The listing builds one solid part. Answer for the finished solid, in the listing's coordinates (mm). A direction names the side the tool comes from. Coordinates: 2 decimals unless noted, no trailing zeros. Write each loop counter-clockwise with the first axis right and the second up, starting at its lowest first coordinate (ties: lowest second). Pieces come first, ordered by that corner, then holes. Notation, with made-up numbers: M -14,-19 L 33,-19 A11 ccw 33,-15 Z; hole C 22,-1.5 d6. An arc over 180 degrees is marked long. Put each result on its own line as item: value. Start each with the question number.
```python
from build123d import *

# Parameters (mm, degrees)
F0_W     = 26
F0_H     = 128
F1_DEPTH = 17
F2_W     = 4
F2_H     = 40
F3_DEPTH = 15
F4_R     = 1


with BuildPart() as f1:
    # F0 (on Top) → F1 (new body)
    with BuildSketch(Plane.XY):
        with Locations((-13, 0)):
            Rectangle(F0_W, F0_H)
    extrude(amount=F1_DEPTH)

    # F2 (on Top) → F3 (cut)
    with BuildSketch(Plane.XY):
        with Locations((-10, 42)):
            Rectangle(F2_W, F2_H)
        with Locations((-4, 42)):
            Rectangle(F2_W, F2_H)
        with Locations((-16, 0)):
            Rectangle(F2_W, F2_H)
        with Locations((-10, 0)):
            Rectangle(F2_W, F2_H)
        with Locations((-4, 0)):
            Rectangle(F2_W, F2_H)
        with Locations((-16, -42)):
            Rectangle(F2_W, F2_H)
        with Locations((-10, -42)):
            Rectangle(F2_W, F2_H)
        with Locations((-4, -42)):
            Rectangle(F2_W, F2_H)
        with Locations((-16, 42)):
            Rectangle(F2_W, F2_H)
        with Locations((-22, 42)):
            Rectangle(F2_W, F2_H)
        with Locations((-22, 0)):
            Rectangle(F2_W, F2_H)
        with Locations((-22, -42)):
            Rectangle(F2_W, F2_H)
    extrude(amount=F3_DEPTH, mode=Mode.SUBTRACT)

    # F4
    f4_edges = [f1.edges().sort_by_distance(p)[0] for p in [
        (-26, 0, 0),
        (-13, -64, 0),
        (0, 0, 0),
        (-13, 64, 0),
        (-26, 64, 8.5),
        (0, 64, 8.5),
        (-26, -64, 8.5),
        (0, -64, 8.5),
    ]]
    fillet(f4_edges, radius=F4_R)


solid = f1.part
```
1) Straight lines are drawn through the part: probe 1 along X at (y, z) = (51, 3.75); probe 2 along Y at (x, z) = (-3.75, 1.5); probe 3 along Z at (x, y) = (-2.75, -2). For each, find the intervals that lie inside material, in ascending order.
2) A cutting plane is placed at B-B on x = -4.75. Write down the section's boundary in (y, z).
3) Given pin 1 Ø1.2 at (x, y) = (-11, -49.5) entering from -Z; pin 2 Ø4.5 at (x, y) = (-4, 8) entering from -Z, each flat-ended and moving along its own axis, determine where each tip first touches the part or whether it passes through.
4) A cutting plane is placed at A-A on y = 53.5. Write down the section's boundary in (x, z).
5) For faces 4 (the face through (-24, -42, 7)), 5 (the face through (-13, 1, 17)), determine the directions among +Z, -Z, +X, -X, +Y, -Y from which every point of the face is accessible in a straight line to the end or side of a thin tool.
6) A cutting plane is placed at C-C on z = 3.25. State how many separate pieces and enclosed holes the cut face has, then the cut area to 3 significant figures.
7) Determine the mould class of faces 1 (the face through (-10, -20, 7)), 2 (the face through (0, -1, 9)), 3 (the face through (-26, -1, 9)) for opening direction X: +X half, -X half, draft (parallel to the pull), parting line (faces both ways), or undercut.
Answers follow:
1. probe 1: x = -26 to -24, -20 to -18, -14 to -12, -8 to -6, -2 to 0
1. probe 2: y = -64 to -62, -22 to -20, 20 to 22, 62 to 64
1. probe 3: z = 15 to 17
2. outline: M -64,1 A1 ccw -63,0 L -62,0 L -62,15 L -22,15 L -22,0 L -20,0 L -20,15 L 20,15 L 20,0 L 22,0 L 22,15 L 62,15 L 62,0 L 63,0 A1 ccw 64,1 L 64,17 L -64,17 Z
3. pin 1: stops at z = 15
3. pin 2: stops at z = 0
4. outline: M -26,1 A1 ccw -25,0 L -24,0 L -24,15 L -20,15 L -20,0 L -18,0 L -18,15 L -14,15 L -14,0 L -12,0 L -12,15 L -8,15 L -8,0 L -6,0 L -6,15 L -2,15 L -2,0 L -1,0 A1 ccw 0,1 L 0,17 L -26,17 Z
5. face 4: -Z
5. face 5: +Z, +X, -X, +Y, -Y
6. separate pieces: 1
6. enclosed holes: 12
6. area: 1,410 mm²
7. face 1: undercut
7. face 2: +X half
7. face 3: -X half
